The listing builds one solid part. Answer for the finished solid, in the listing's coordinates (mm). Round coordinates to 2 decimals unless told otherwise and drop trailing zeros. Loops run counter-clockwise (first coordinate to the right, second up) from the corner with the lowest first, then second, coordinate; pieces in that order, holes last. Notation, with made-up numbers: (36, 42.25) -> (43, 42.25) arc R16 ccw to (43, 68.25) -> close; hole circle Ø3 at (71, 24.5). An arc over 180 degrees is marked (long way). Use a Markdown table: item, result. Add a question column.
Q1. Section B-B on x = 41.5 is taken. Give the vertices of the cut face in (y, z).
Q2. Given pin 1 Ø1 at (y, z) = (24.5, 1) entering from +X; pin 2 Ø3 at (y, z) = (21.5, 1) entering from -X (3 decimals); pin 3 Ø3 at (y, z) = (59, 1.5) entering from -X, each flat-ended and moving along its own axis, determine where each tip first touches the part or whether it passes through.
Q3. Section D-D on y = 54.5 is taken. Give the vertices of the cut face in (x, z).
Q4. Section C-C on z = 4.45 is taken. Give the vertices of the cut face in (x, y), then the cut area to 3 significant figures.
Q5. Consider line 1 (X direction, y = 26.5, z = 1); line 2 (X direction, y = 20, z = 0.3); line 3 (Y direction, x = 9, z = 4). Determine where each line is inside the solid, lowest interval first.
Q6. Section A-A on y = 33 is taken. Give the vertices of the cut face in (x, z), then the cut area to 3 significant figures.
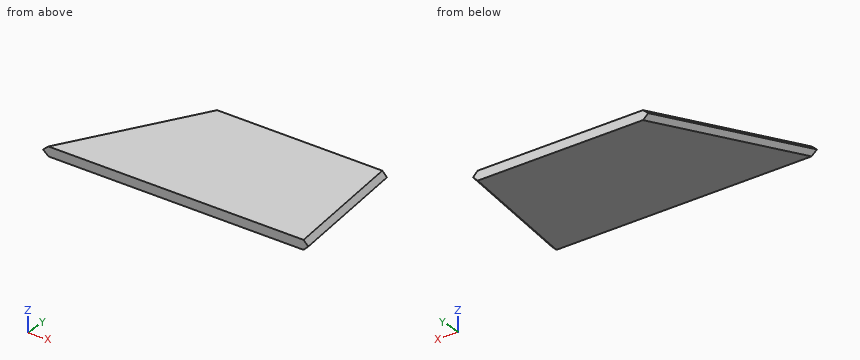
from build123d import *

# Parameters (mm, degrees)
BOSS_EXTRUDE1_DEPTH = 5.2832
CHAMFER3_SIZE       = 3.81


with BuildPart() as part:
    # Sketch2 → Boss-Extrude1 (new body)
    with BuildSketch(Plane.XY):
        Polygon((0, 0), (152.4, 0), (144.78, 71.882), (43.18, 71.882), align=None)
    extrude(amount=BOSS_EXTRUDE1_DEPTH)

    # Chamfer3
    # the kernel refuses this chamfer: 3.81 mm, written as the material it takes off along each edge
    with BuildSketch(Plane(origin=(153.432881845, -9.743518742, 5.2832), x_dir=(0.027342674184069608, 0.002898516697957921, -0.9996219169112969), z_dir=(-0.10541641348659767, 0.9944281672235671, 0))) as chamfer3_piece_1:
        Polygon((CHAMFER3_SIZE * 0.999621916911, CHAMFER3_SIZE * 0.0274958766106), (-CHAMFER3_SIZE * 0.0274958766106, CHAMFER3_SIZE * 0.999621916911), (0, 0), align=None)
    extrude(amount=91.880982955, mode=Mode.SUBTRACT)
    with BuildSketch(Plane(origin=(153.432881845, -9.743518742, 0), x_dir=(0.027342674184069608, 0.002898516697957921, 0.9996219169112969), z_dir=(-0.10541641348659767, 0.9944281672235671, 0))) as chamfer3_piece_2:
        Polygon((CHAMFER3_SIZE * 0.999621916911, -CHAMFER3_SIZE * 0.0274958766106), (-CHAMFER3_SIZE * 0.0274958766106, -CHAMFER3_SIZE * 0.999621916911), (0, 0), align=None)
    extrude(amount=91.880982955, mode=Mode.SUBTRACT)
    with BuildSketch(Plane(origin=(48.225451027, 80.281192003, 5.2832), x_dir=(-0.023570167662218693, 0.014158757959636668, -0.9996219169112966), z_dir=(-0.514941136817021, -0.8572255395248057, 0))) as chamfer3_piece_3:
        Polygon((CHAMFER3_SIZE * 0.999621916911, CHAMFER3_SIZE * 0.0274958766106), (-CHAMFER3_SIZE * 0.0274958766106, CHAMFER3_SIZE * 0.999621916911), (0, 0), align=None)
    extrude(amount=103.450468888, mode=Mode.SUBTRACT)
    with BuildSketch(Plane(origin=(48.225451027, 80.281192003, 0), x_dir=(-0.023570167662218693, 0.014158757959636668, 0.9996219169112966), z_dir=(-0.514941136817021, -0.8572255395248057, 0))) as chamfer3_piece_4:
        Polygon((CHAMFER3_SIZE * 0.999621916911, -CHAMFER3_SIZE * 0.0274958766106), (-CHAMFER3_SIZE * 0.0274958766106, -CHAMFER3_SIZE * 0.999621916911), (0, 0), align=None)
    extrude(amount=103.450468888, mode=Mode.SUBTRACT)


solid = part.part
Checked values:
| question | item | result |
|---|---|---|
| 1 | outline | (0, 0) -> (61.69, 0) -> (66.82, 2.64) -> (61.69, 5.28) -> (0, 5.28) -> close |
| 2 | pin 1 | stops at x = 147.48 |
| 2 | pin 2 | stops at x = 14.225 |
| 2 | pin 3 | stops at x = 36.22 |
| 3 | outline | (34.1, 2.64) -> (37.18, 0) -> (142.79, 0) -> (145.45, 2.64) -> (142.79, 5.28) -> (37.18, 5.28) -> close |
| 4 | outline | (3.47, 0) -> (149.41, 0) -> (141.79, 71.88) -> (46.65, 71.88) -> close |
| 4 | area | 8,660 mm2 |
| 5 | line 1 | x = 19.2 to 146.77 |
| 5 | line 2 | x = 16.11 to 146.75 |
| 5 | line 3 | y = 0 to 10.08 |
| 6 | outline | (21.19, 2.64) -> (24.27, 0) -> (145.07, 0) -> (147.73, 2.64) -> (145.07, 5.28) -> (24.27, 5.28) -> close |
| 6 | area | 653 mm2 |
